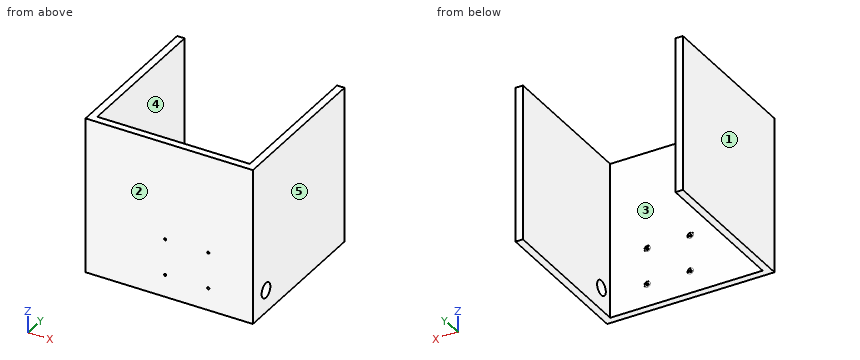
```python
from build123d import *

# Parameters (mm, degrees)
EXTRUDE_2_DEPTH                = 210
SKETCH_3_R                     = 10
CUT_EXTRUDE_1_DEPTH            = 10
HOLE_WIZARD_M2_5_1_D           = 2.9
HOLE_WIZARD_M2_5_1_CBORE_D     = 8
HOLE_WIZARD_M2_5_1_CBORE_DEPTH = 0.5


with BuildPart() as part:
    # 草图2 → 凸台-拉伸2 (new body)
    with BuildSketch(Plane.XY):
        Polygon((0, 0), (225, 0), (225, 210), (215, 210), (215, 10), (10, 10), (10, 210), (0, 210), align=None)
    extrude(amount=-EXTRUDE_2_DEPTH)

    # 草图3 → 切除-拉伸1 (cut)
    with BuildSketch(Plane(origin=(225, 0, 0), x_dir=(0, 0, -1), z_dir=(1, 0, 0))):
        with Locations((180, 30)):
            Circle(SKETCH_3_R)
    extrude(amount=-CUT_EXTRUDE_1_DEPTH, mode=Mode.SUBTRACT)

    # M2.5 六角头螺栓的柱形沉头孔1 (through all)
    with Locations(Plane(origin=(0, 10, 0), x_dir=(1, 0, 0), z_dir=(0, 1, 0))):
        with Locations((107, 180), (107, 131.4), (165, 131.4), (165, 180)):
            CounterBoreHole(HOLE_WIZARD_M2_5_1_D / 2, HOLE_WIZARD_M2_5_1_CBORE_D / 2, HOLE_WIZARD_M2_5_1_CBORE_DEPTH)


solid = part.part
```
Here's how the part is built. I have some questions about the finished solid (model axes, mm). Face numbers are marked on the shaded views. A direction names the side the tool comes from. Round coordinates to 2 decimals unless told otherwise and drop trailing zeros. Write each loop counter-clockwise with the first axis right and the second up, starting at its lowest first coordinate (ties: lowest second). Pieces come first, ordered by that corner, then holes. Notation, with made-up numbers: M -26.75,-20.75 L 14.25,-20.75 A29 ccw 14.25,0.25 Z; hole C 78.5,-32 d2. An arc over 180 degrees is marked long. Answer as CSV lines item,"result". Start each with the question number.
1. Suppose I cut it at D-D on z = -25. Write out the boundary of the cut face in (x, y).
2. I'm going to push flat-ended pins straight in: pin 1 Ø2.5 at (x, z) = (166, -182) entering from +Y; pin 2 Ø9 at (x, z) = (164, -130.5) entering from +Y. Where does each tip first touch, or does it pass through?
3. Suppose I cut it at B-B on y = 30. Write out the boundary of the cut face in (x, z), then the cut area to 3 significant figures.
4. I need wall thicknesses on probe 1 along Z at (x, y) = (165, 9); probe 2 along X at (y, z) = (9, -180); probe 3 along Z at (x, y) = (107, 9.75). Which ranges of each line are inside material? Lowest first, please.
5. Suppose I cut it at A-A on y = 165.5. Write out the boundary of the cut face in (x, z).
6. On a 3-axis mill with a long thin cutter (end or side, diameter ignored), from which of +Z, -Z, +X, -X, +Y, -Y can I reach the whole of each face in a straight line? I mean the marked faces 4 and 5. Say none if no direction works.
7. Suppose I cut it at C-C on z = -173. Write out the boundary of the cut face in (x, y), then the cut area to 3 significant figures.
8. Thinking about a two-plate mould opening in X: for the marked faces 1, 2 and 3, which applies, released by +X, released by -X, zero draft, split by the parting line, or undercut?
Check result:
1,outline,"M 0,0 L 225,0 L 225,210 L 215,210 L 215,10 L 10,10 L 10,210 L 0,210 Z"
2,pin 1,"stops at y = 9.5"
2,pin 2,"stops at y = 10"
3,outline,"M 0,-210 L 10,-210 L 10,0 L 0,0 Z; M 215,-210 L 225,-210 L 225,-190 L 215,-190 Z; M 215,-170 L 225,-170 L 225,0 L 215,0 Z"
3,area,"4,000 mm2"
4,probe 1,"z = -210 to -181.45, -178.55 to -132.85, -129.95 to 0"
4,probe 2,"x = 0 to 105.55, 108.45 to 163.55, 166.45 to 225"
4,probe 3,"z = -210 to -184, -176 to -135.4, -127.4 to 0"
5,outline,"M 0,-210 L 10,-210 L 10,0 L 0,0 Z; M 215,-210 L 225,-210 L 225,0 L 215,0 Z"
6,face 4,"+Z, -Z, +Y"
6,face 5,"+Z, -Z, +X, +Y, -Y"
7,outline,"M 0,0 L 225,0 L 225,22.86 L 215,22.86 L 215,10 L 10,10 L 10,210 L 0,210 Z; M 215,37.14 L 225,37.14 L 225,210 L 215,210 Z"
7,area,"6,110 mm2"
8,face 1,"released by -X"
8,face 2,"zero draft"
8,face 3,"undercut"
